Geometry check sheet. Reference: the model listing, model coordinates, mm. A direction names the side the tool comes from. Coordinates: 2 decimals unless noted, no trailing zeros. Order: outer loops, then holes, each group sorted by start corner. A loop starts at its lowest first (then second) coordinate and runs counter-clockwise, first axis right, second up. Notation, with made-up numbers: (-2.75, 85.25) - (38.25, 85.25) arc R33 ccw to (38.25, 117.25) - close; hole circle Ø5 at (20, 84.25). An arc over 180 degrees is marked (long way). Return JSON: item names as keys, results as strings. Group by question number.
Item 1: Scan lines: probe 1 along Y at (x, z) = (-15, 2.1); probe 2 along Y at (x, z) = (5.5, -7.5); probe 3 along Z at (x, y) = (-15, -26). Record each from-to range of solid material in increasing order.
Item 2: Section check B-B on z = -3. Enter the section's corners in (x, y).
Item 3: Draft check along Y on faces 6 (the cylindrical face through (17.32, -27.46, -7.87)), 7 (the flat face through (-20, 3, 0)). Enter one of: pulls with the +Y half, pulls with the -Y half, needs draft (parallel to the pull), parting line crosses it, or undercut.
Item 4: Section check A-A on x = -15. Enter the section's corners in (y, z).
Item 5: Gauge pin test, flat ends, axial feed: pin 1 (10 mm diameter, centred on y = -6, z = -14.5, fed in from -X); pin 2 (5.5 mm diameter, centred on x = 6.5, y = -27, fed in from -Z); pin 3 (5 mm diameter, centred on y = -8.5, z = -15, fed in from +X). Record the tip position at first contact, or that the pin passes through.
Item 6: Section check C-C on y = -13. Enter the section's corners in (x, z).
Item 7: Section check D-D on z = -16.75. Enter the section's corners in (x, y), then the cut area to 3 significant figures.
Item 8: Tool access check on faces 1 (the flat face through (-15, -7.7, 3)), 2 (the flat face through (19, -25, -10)), 3 (the flat face through (19.15, -28, 3)), 4 (the flat face through (-20, -25, -10)), 5 (the flat face through (0.04, -9.72, -13.1)). Record the directions out of +Z, -Z, +X, -X, +Y, -Y that give a thin tool (end or side, any length) a straight path to the whole face; none if there is none.
from build123d import *

# Parameters (mm, degrees)
F0_W           = 60
F0_H           = 60
F0_R           = 3.15
F1_DEPTH       = 4
F2_W           = 8.3
F2_H           = 4.5
F2_H_2         = 4
F3_DEPTH       = 2.8
F4_W           = 26
F4_H           = 24
F5_DEPTH       = 24
F6_R           = 3.05
F7_DEPTH       = 43.001
F8_W           = 60
F8_H           = 5
F9_DEPTH       = 20
F11_DEPTH      = 3
F11_DEPTH_BACK = 3
F12_R          = 3.15
F13_DEPTH      = 5.001


with BuildPart() as f1:
    # F0 (on Top) → F1 (new body)
    with BuildSketch(Plane.XY):
        Rectangle(F0_W, F0_H)
        with Locations((-15, -13)):
            Circle(F0_R, mode=Mode.SUBTRACT)
        with Locations((15, -13)):
            Circle(F0_R, mode=Mode.SUBTRACT)
    extrude(amount=F1_DEPTH)

    # F2 (on face) → F3 (cut)
    with BuildSketch(Plane.XY.offset(4)):
        with Locations((-15, -27.75)):
            Rectangle(F2_W, F2_H)
        with Locations((15, -27.75)):
            Rectangle(F2_W, F2_H)
        with Locations((-15, -5.7)):
            Rectangle(F2_W, F2_H_2)
        with Locations((15, -5.7)):
            Rectangle(F2_W, F2_H_2)
    extrude(amount=-F3_DEPTH, mode=Mode.SUBTRACT)

    # F4 (on face) → F5 (join)
    with BuildSketch(Plane(origin=(0, 0, 0), x_dir=(1, 0, 0), z_dir=(0, 0, -1))):
        with Locations((0, -18)):
            Rectangle(F4_W, F4_H)
    extrude(amount=F5_DEPTH)

    # F6 (on face) → F7 (cut, through all)
    with BuildSketch(Plane.YZ.offset(13)):
        with BuildLine():
            ThreePointArc((30, -12), (26.485281, -20.485281), (18, -24))
            Line((18, -24), (30, -24))
            Line((30, -24), (30, -12))
        make_face()
        with BuildLine():
            ThreePointArc((18, -24), (9.514719, -20.485281), (6, -12))
            Line((6, -12), (6, -24))
            Line((6, -24), (18, -24))
        make_face()
        with Locations((18, -12)):
            Circle(F6_R)
    extrude(amount=-F7_DEPTH, mode=Mode.SUBTRACT)

    # F8 (on face) → F9 (join)
    with BuildSketch(Plane(origin=(0, 0, 0), x_dir=(1, 0, 0), z_dir=(0, 0, -1))):
        with Locations((0, 27.5)):
            Rectangle(F8_W, F8_H)
    extrude(amount=F9_DEPTH)

    # F10 (on Right) → F11 (join, two sides)
    with BuildSketch(Plane.YZ) as f11_sk:
        Polygon((-25, 0), (-25, -20), (6, -6), (6, 0), align=None)
    extrude(amount=F11_DEPTH)
    extrude(f11_sk.sketch, amount=-F11_DEPTH_BACK)

    # F12 (on face) → F13 (cut, through all)
    with BuildSketch(Plane(origin=(0, -25, 0), x_dir=(-1, 0, 0), z_dir=(0, 1, 0))):
        with Locations((15, -10)):
            Circle(F12_R)
        with Locations((-15, -10)):
            Circle(F12_R)
    extrude(amount=-F13_DEPTH, mode=Mode.SUBTRACT)


solid = f1.part
Computed:
{
 "1": {"probe 1": "y = -25.5 to -16.15, -9.85 to -7.7, -3.7 to 30", "probe 2": "y = -30 to -25, 6 to 30", "probe 3": "z = -20 to -13.15, -6.85 to 1.2"},
 "2": {"outline": "(-30, -30) - (30, -30) - (30, -25) - (3, -25) - (3, 6) - (13, 6) - (13, 30) - (-13, 30) - (-13, 6) - (-3, 6) - (-3, -25) - (-30, -25) - close"},
 "3": {"face 6": "needs draft", "face 7": "undercut"},
 "4": {"outline": "(-30, -20) - (-25, -20) - (-25, -13.15) - (-30, -13.15) - close; (-30, -6.85) - (-25, -6.85) - (-25, 0) - (-16.15, 0) - (-16.15, 4) - (-25.5, 4) - (-25.5, 1.2) - (-30, 1.2) - close; (-9.85, 0) - (30, 0) - (30, 4) - (-3.7, 4) - (-3.7, 1.2) - (-7.7, 1.2) - (-7.7, 4) - (-9.85, 4) - close"},
 "5": {"pin 1": "stops at x = -3", "pin 2": "stops at z = -20", "pin 3": "stops at x = 3"},
 "6": {"outline": "(-30, 0) - (-18.15, 0) - (-18.15, 4) - (-30, 4) - close; (-11.85, 0) - (-3, 0) - (-3, -14.58) - (3, -14.58) - (3, 0) - (11.85, 0) - (11.85, 4) - (-11.85, 4) - close; (18.15, 0) - (30, 0) - (30, 4) - (18.15, 4) - close"},
 "7": {"outline": "(-30, -30) - (30, -30) - (30, -25) - (3, -25) - (3, -17.8) - (-3, -17.8) - (-3, -25) - (-30, -25) - close; (-13, 6.98) - (13, 6.98) - (13, 29.02) - (-13, 29.02) - close", "area": "916 mm²"},
 "8": {"face 1": "+Z", "face 2": "-Z, +X", "face 3": "+Z, -Y", "face 4": "-Z, -X", "face 5": "-Z, +X, -X"}
}
